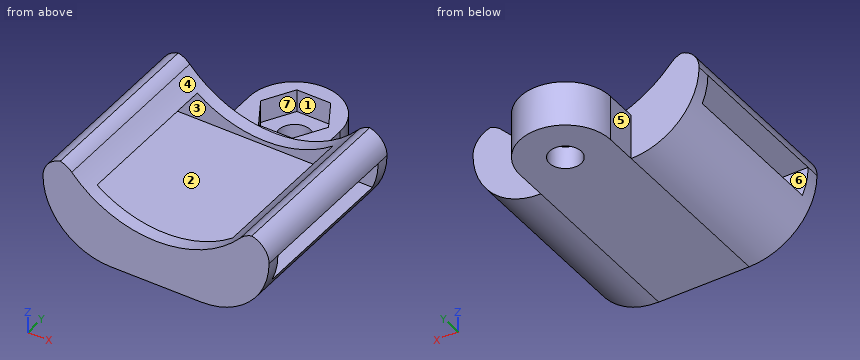
from build123d import *
from build123d.topology import SkipClean

# Parameters (mm, degrees)
ESBO_O1_R                = 1.75
ESBO_O1_W                = 25
ESBO_O1_H                = 20
RESSALTO_EXTRUS_O1_DEPTH = 2.5
RESSALTO_EXTRUS_O2_DEPTH = 20
ESBO_O4_W                = 3
ESBO_O4_H                = 17
CORTE_EXTRUS_O1_DEPTH    = 39
FILETE1_R                = 7.5
FILETE2_R                = 2.5
RESSALTO_EXTRUS_O3_DEPTH = 2.5


with BuildPart() as part:
    # Esboço1 → Ressalto-extrusão1 (new body)
    # profile 1 of 2: a face of its own
    with BuildSketch(Plane.XY):
        with BuildLine():
            Line((5, 0), (5, -3.5))
            Line((5, -3.5), (-5, -3.5))
            Line((-5, -3.5), (-5, 0))
            ThreePointArc((-5, 0), (0, 5), (5, 0))
        make_face()
        Circle(ESBO_O1_R, mode=Mode.SUBTRACT)
    # profile 2 of 2: a face of its own
    with BuildSketch(Plane.XY):
        with Locations((0, -13.5)):
            Rectangle(ESBO_O1_W, ESBO_O1_H)
    extrude(amount=RESSALTO_EXTRUS_O1_DEPTH)

    # Esboço3 → Ressalto-extrusão2 (add)
    with BuildSketch(Plane.XZ.offset(23.5)):
        with BuildLine():
            Line((12.5, 10), (10, 10))
            ThreePointArc((10, 10), (0, 5), (-10, 10))
            Line((-10, 10), (-12.5, 10))
            Line((-12.5, 10), (-12.5, 2.5))
            Line((-12.5, 2.5), (12.5, 2.5))
            Line((12.5, 2.5), (12.5, 10))
        make_face()
    extrude(amount=-RESSALTO_EXTRUS_O2_DEPTH)

    # Esboço4 → Corte-extrusão1 (cut)
    with BuildSketch(Plane.ZY.offset(12.5)):
        with Locations((6, -13.5)):
            Rectangle(ESBO_O4_W, ESBO_O4_H)
    extrude(amount=-CORTE_EXTRUS_O1_DEPTH, mode=Mode.SUBTRACT)

    # Filete1
    # the kernel refuses this fillet: 7.5 mm, written as the material it takes off along each edge
    with BuildSketch(Plane(origin=(-12.5, -42.25, 0), x_dir=(1, 0, 0), z_dir=(0, 1, 0)), Plane(origin=(12.5, 15.25, 0), x_dir=(-1, 0, 0), z_dir=(0, -1, 0))) as filete1_piece_1:
        with BuildLine():
            CenterArc((FILETE1_R, -FILETE1_R), FILETE1_R, 90, 90)
            Line((0, -FILETE1_R), (0, 0))
            Line((0, 0), (FILETE1_R, 0))
        make_face()
    extrude(amount=57.5, mode=Mode.SUBTRACT)

    # Filete2
    # the kernel refuses this fillet: 2.5 mm, written as the material it takes off along each edge
    with BuildSketch(Plane(origin=(10, -26.450849719, 10), x_dir=(1, 0, 0), z_dir=(0, 1, 0))) as filete2_piece_1:
        with BuildLine():
            CenterArc((1.180339887, 2.5), FILETE2_R, 221.810314896, 48.189685104)
            ThreePointArc((-0.683050094, 0.833333333), (-0.332541723, 0.424029939), (0, 0))
            Line((0, 0), (1.180339887, 0))
        make_face()
    extrude(amount=25.901699437, mode=Mode.SUBTRACT)
    with BuildSketch(Plane(origin=(-10, -26.450849719, 10), x_dir=(0.6339223950926707, 0, -0.7733966621339738), z_dir=(0, 1, 0))) as filete2_piece_2:
        with BuildLine():
            CenterArc((1.185247767, 2.497676917), FILETE2_R, 219.340106271, 48.189685104)
            Line((-0.748243889, 0.912870929), (0, 0))
            ThreePointArc((0, 0), (0.538748985, 0.011615415), (1.07749797, 0))
        make_face()
    extrude(amount=25.901699437, mode=Mode.SUBTRACT)
    with BuildSketch(Plane(origin=(12.5, -29.75, 10), x_dir=(0, 0, -1), z_dir=(0, 1, 0)), Plane(origin=(-12.5, -29.75, 10), x_dir=(1, 0, 0), z_dir=(0, 1, 0))) as filete2_piece_3:
        with BuildLine():
            CenterArc((FILETE2_R, FILETE2_R), FILETE2_R, 180, 90)
            Line((0, FILETE2_R), (0, 0))
            Line((0, 0), (FILETE2_R, 0))
        make_face()
    extrude(amount=32.5, mode=Mode.SUBTRACT)

    # Esboço5 → Ressalto-extrusão3 (add)
    # profile 1 of 6: a face of its own
    with SkipClean():  # the faces are left unmerged after this step: merging them gives an invalid solid
        with BuildSketch(Plane.XY.offset(2.5)):
            with BuildLine():
                ThreePointArc((-3.570714214, -3.5), (-4.628907596, -1.890294809), (-5, 0))
                Line((-5, 0), (-5, -3.5))
                Line((-5, -3.5), (-3.570714214, -3.5))
            make_face()
        # profile 2 of 6: a face of its own
        with BuildSketch(Plane.XY.offset(2.5)):
            with BuildLine():
                Line((5, -3.5), (5, 0))
                ThreePointArc((5, 0), (4.628907596, -1.890294809), (3.570714214, -3.5))
                Line((3.570714214, -3.5), (5, -3.5))
            make_face()
        # profile 3 of 6: a face of its own
        with BuildSketch(Plane.XY.offset(2.5)):
            with BuildLine():
                Line((5, -5), (5, -3.5))
                Line((5, -3.5), (3.570714214, -3.5))
                ThreePointArc((3.570714214, -3.5), (1.936491652, -4.609772238), (-4.7e-08, -5))
                Line((-4.7e-08, -5), (5, -5))
            make_face()
        # profile 4 of 6: a face of its own
        with BuildSketch(Plane.XY.offset(2.5)):
            with BuildLine():
                Line((-3.570714214, -3.5), (-5, -3.5))
                Line((-5, -3.5), (-5, -5))
                Line((-5, -5), (-4.7e-08, -5))
                ThreePointArc((-4.7e-08, -5), (-1.936491695, -4.60977222), (-3.570714214, -3.5))
            make_face()
        # profile 5 of 6: a face of its own
        with BuildSketch(Plane.XY.offset(2.5)):
            with BuildLine():
                Line((3.570714214, -3.5), (-3.570714214, -3.5))
                ThreePointArc((-3.570714214, -3.5), (-1.936491695, -4.60977222), (-4.7e-08, -5))
                ThreePointArc((-4.7e-08, -5), (1.936491652, -4.609772238), (3.570714214, -3.5))
            make_face()
        # profile 6 of 6: a face of its own
        with BuildSketch(Plane.XY.offset(2.5)):
            with BuildLine():
                ThreePointArc((5, 0), (0, 5), (-5, 0))
                ThreePointArc((-5, 0), (-4.628907596, -1.890294809), (-3.570714214, -3.5))
                Line((-3.570714214, -3.5), (3.570714214, -3.5))
                ThreePointArc((3.570714214, -3.5), (4.628907596, -1.890294809), (5, 0))
            make_face()
            Polygon((1.876388375, 3.25), (3.75277675, 0), (1.876388375, -3.25), (-1.876388375, -3.25), (-3.75277675, 0), (-1.876388375, 3.25), align=None, mode=Mode.SUBTRACT)
        extrude(amount=RESSALTO_EXTRUS_O3_DEPTH)


solid = part.part
Could you check a few things on this model? Use its own coordinates, in mm. Face numbers are marked on the shaded views. A direction names the side the tool comes from. Round coordinates to 2 decimals unless told otherwise and drop trailing zeros. Write each loop counter-clockwise with the first axis right and the second up, starting at its lowest first coordinate (ties: lowest second). Pieces come first, ordered by that corner, then holes. Notation, with made-up numbers: (89, 65) - (132, 65) arc R4 cw to (132, 69) - close; hole circle Ø5 at (-30.75, 68.5). An arc over 180 degrees is marked (long way). Put each result on its own line as item: value. Start each with the question number.
(1) Will these pins go through, and if not, where does the flat tip stop? pin 1 (3.5 mm diameter, centred on x = -1.5, z = 5.5, fed in from +Y); pin 2 (2.5 mm diameter, centred on x = 9, y = -12, fed in from -Z); pin 3 (4 mm diameter, centred on y = -2.5, z = 2.5, fed in from -X); pin 4 (5 mm diameter, centred on x = 0.5, y = -1.5, fed in from +Z).
(2) I want a section at B-B, the plane z = 8.25. Please give me the cut outline in (x, y).
(3) For the marked faces 5, 6 and 7, which set-ups out of +Z, -Z, +X, -X, +Y, -Y let a thin tool reach every point of the face, with its end or its side?
(4) I want a section at A-A, the plane y = -5.5. Please give me the cut outline in (x, z), plus the area to 3 significant figures.
(5) I need wall thicknesses on probe 1 along Y at (x, z) = (0, 1.6); probe 2 along Y at (x, z) = (8.5, 5.25); probe 3 along Z at (x, y) = (-4.5, -12.5). Which ranges of each line are inside material? Lowest first, please.
(6) I want a section at C-C, the plane z = 3.75. Please give me the cut outline in (x, y), plus the area to 3 significant figures.
(7) I want a section at D-D, the plane z = 2. Please give me the cut outline in (x, y), plus the area to 3 significant figures.
(8) Thinking about a two-plate mould opening in Z: for the marked faces 1, 2, 3 and 4, which applies, released by +Z, released by -Z, zero draft, split by the parting line, or undercut?
Here are the results:
1. pin 1: stops at y = 5
1. pin 2: stops at z = 0.52
1. pin 3: stops at x = -11.75
1. pin 4: stops at z = 5.16
2. outline: (-12.38, -23.5) - (-8.41, -23.5) - (-8.41, -3.5) - (-12.38, -3.5) - close; (8.41, -23.5) - (12.38, -23.5) - (12.38, -3.5) - (8.41, -3.5) - close
3. face 5: +Z, -Z, -X, +Y
3. face 6: +X, -X
3. face 7: +Z
4. outline: (-12.5, 7.5) - (-7.5, 7.5) arc R12.5 cw to (-9.32, 9.17) arc R2.5 ccw to (-10.59, 9.93) arc R2.5 ccw to start; (-11.87, 4.5) arc R7.5 ccw to (-5, 0) - (5, 0) arc R7.5 ccw to (11.87, 4.5) - close; (7.5, 7.5) - (12.5, 7.5) arc R2.5 ccw to (10.59, 9.93) arc R2.5 ccw to (9.32, 9.17) arc R12.5 cw to start
4. area: 105 mm^2
5. probe 1: y = -23.5 to -1.75, 1.75 to 5
5. probe 2: y = -23.5 to -22, -5 to -3.5
5. probe 3: z = 0 to 4.5
6. outline: (-11.5, -23.5) - (11.5, -23.5) - (11.5, -3.5) - (5, -3.5) - (5, 0) arc R5 ccw to (-5, 0) - (-5, -3.5) - (-11.5, -3.5) - close; hole (-3.75, 0) - (-1.88, -3.25) - (1.88, -3.25) - (3.75, 0) - (1.88, 3.25) - (-1.88, 3.25) - close
6. area: 497 mm^2
7. outline: (-10.1, -23.5) - (10.1, -23.5) - (10.1, -3.5) - (5, -3.5) - (5, 0) arc R5 ccw to (-5, 0) - (-5, -3.5) - (-10.1, -3.5) - close; hole circle Ø3.5 at (0, 0)
7. area: 469 mm^2
8. face 1: zero draft
8. face 2: undercut
8. face 3: undercut
8. face 4: released by +Z
